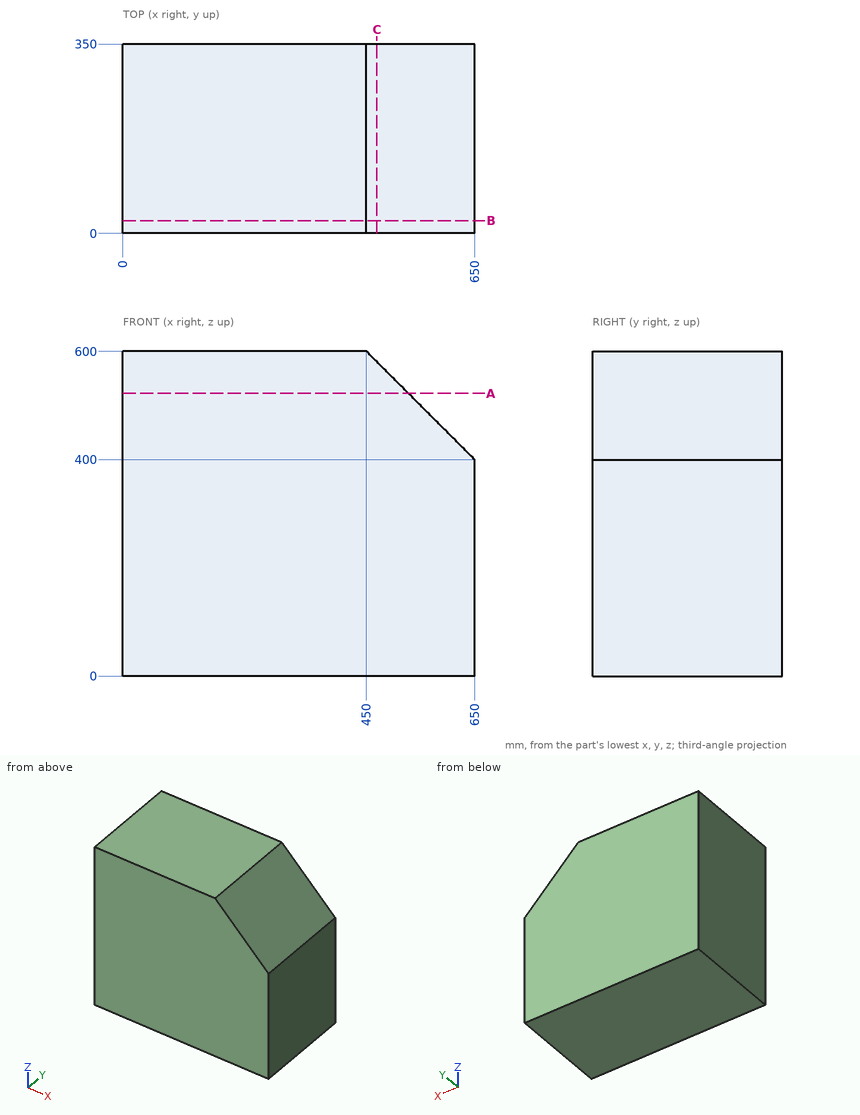
Answer from the drawing. Dimensions are ordinates in mm from the lowest x, y and z of the part. Round coordinates to 2 decimals unless told otherwise and drop trailing zeros. Write each loop counter-clockwise with the first axis right and the second up, starting at its lowest first coordinate (ties: lowest second). Pieces come first, ordered by that corner, then holes. Notation, with made-up numbers: M -23,43.5 L 36,43.5 A31 ccw 36,72.5 Z; hole C 9.5,-38.5 d4. An arc over 180 degrees is marked long. Write each question's results on one line, items separated by ' | '. Start each with the question number.
Item 1: Find section B-B on y = 23.5. Write down the section's boundary in (x, z).
Item 2: Straight lines are drawn through the part: probe 1 along X at (y, z) = (49, 497); probe 2 along X at (y, z) = (292, 419.5); probe 3 along Z at (x, y) = (571, 276). For each, find the intervals that lie inside material, in ascending order.
Item 3: Find section A-A on z = 522.5. Write down the section's boundary in (x, y).
Item 4: Find section C-C on x = 469.5. Write down the section's boundary in (y, z).
Item 5: Given pin 1 Ø3 at (x, y) = (456, 297.5) entering from +Z, flat-ended and moving along its own axis, determine where the tip first touches the part or whether it passes through.
Answer block:
1) outline: M 0,0 L 650,0 L 650,400 L 450,600 L 0,600 Z
2) probe 1: x = 0 to 553 | probe 2: x = 0 to 630.5 | probe 3: z = 0 to 479
3) outline: M 0,0 L 527.5,0 L 527.5,350 L 0,350 Z
4) outline: M 0,0 L 350,0 L 350,580.5 L 0,580.5 Z
5) pin 1: stops at z = 595.5
